```python
from build123d import *

# Parameters (mm, degrees)
BOSS_EXTRUDE1_DEPTH = 10
SKETCH4_R           = 2.5
CUT_EXTRUDE1_DEPTH  = 5
SKETCH5_R           = 2.5
CUT_EXTRUDE2_DEPTH  = 5


with BuildPart() as part:
    # 3DSketch1 → Boss-Extrude1 (new body)
    with BuildSketch(Plane(origin=(0, 0, 0), x_dir=(0.8320502943378437, 0.554700196225229, 0), z_dir=(0, 0, -1))):
        Polygon((0, 0), (8.320502943, 5.547001962), (13.867504906, -2.773500981), (18.027756377, 0), (9.707253434, 12.480754415), (-2.773500981, 4.160251472), align=None)
    extrude(amount=-BOSS_EXTRUDE1_DEPTH)

    # Sketch4 → Cut-Extrude1 (cut)
    with BuildSketch(Plane.ZY.offset(-10)):
        with Locations((5, 5)):
            Circle(SKETCH4_R)
    extrude(amount=-CUT_EXTRUDE1_DEPTH, mode=Mode.SUBTRACT)

    # Sketch5 → Cut-Extrude2 (cut)
    with BuildSketch(Plane(origin=(0, 0, 0), x_dir=(1, 0, 0), z_dir=(0, 1, 0))):
        with Locations(Location((5, -5, 0), (0, 0, 270))):
            Circle(SKETCH5_R)
    extrude(amount=-CUT_EXTRUDE2_DEPTH, mode=Mode.SUBTRACT)


solid = part.part
```
Input: part model. Units: mm. Frame: model coordinates. A direction names the side the tool comes from. Give positions to 0.01 mm unless a question says otherwise; leave off trailing zeros. Write each loop counter-clockwise with the first axis right and the second up, starting at its lowest first coordinate (ties: lowest second). Pieces come first, ordered by that corner, then holes. Notation, with made-up numbers: (31, -4) - (64, -4) arc R26 cw to (64, 28) - close; hole circle Ø6 at (-39.5, -29). An arc over 180 degrees is marked (long way). Write item = value, one per line. Start each with the question number.
1. First-contact query: pin 1 Ø5 at (y, z) = (4, 7) entering from -X; pin 2 Ø2 at (x, z) = (6.5, 3.5) entering from +Y; pin 3 Ø6 at (y, z) = (5, 5) entering from +X. Flat tips, straight axial feed; report the tip coordinate or a pass-through.
2. Section query B-B, the plane z = 5. Output: boundary loops of the cut face in (x, y), then the cut area to 3 significant figures.
3. Section query A-A, the plane x = 3. Output: boundary loops of the cut face in (y, z).
4. Section query C-C, the plane y = -2.25. Output: boundary loops of the cut face in (x, z), then the cut area to 3 significant figures.
5. Mould query, pull axis Z, two halves, no side actions, for faces 3 (the cylindrical face through (5.751, -2.465, 7.385)), 4 (the flat face through (12, 10, 5)), 5 (the cylindrical face through (12.465, 5.751, 7.385)), 6 (the flat face through (11, 1, 10)). Classes: released by +Z, released by -Z, zero draft, split by the parting line, or undercut.
6. Ray query, L1, parallel to X at y = -1.4, z = 5; L2, parallel to Y at x = 12.05, z = 5; L3, parallel to X at y = 8, z = 8.25. Return the intervals inside material, ascending.
7. Section query D-D, the plane y = 5. Output: boundary loops of the cut face in (x, z).
8. Access query for faces 1 (the flat face through (3, 0, 3)), 2 (the flat face through (0, -3, 5)). Directions: +Z, -Z, +X, -X, +Y, -Y. A direction counts if a zero-diameter tool reaches every point of the face in a straight line with its end or side. Return the directions, or none.
Check sheet entries:
q1.pin_1 = 10
q1.pin_2 = 0
q1.pin_3 = 15
q2.outline = (0, -5) - (2.5, -5) - (2.5, 0) - (0, 0) - close; (7.5, -5) - (15, -5) - (15, 2.5) - (10, 2.5) - (10, 0) - (7.5, 0) - close; (10, 7.5) - (15, 7.5) - (15, 10) - (10, 10) - close
q2.area = 75.0 mm2
q3.outline = (-5, 0) - (0, 0) - (0, 3.5) - (-5, 3.5) - close; (-5, 6.5) - (0, 6.5) - (0, 10) - (-5, 10) - close
q4.outline = (0, 0) - (15, 0) - (15, 10) - (0, 10) - close; hole circle Ø5 at (5, 5)
q4.area = 130 mm2
q5.face_3 = undercut
q5.face_4 = zero draft
q5.face_5 = undercut
q5.face_6 = released by +Z
q6.L1 = 0 to 2.5, 7.5 to 15
q6.L2 = -5 to 2.5, 7.5 to 10
q6.L3 = 10 to 15
q7.outline = (10, 0) - (15, 0) - (15, 2.5) - (10, 2.5) - close; (10, 7.5) - (15, 7.5) - (15, 10) - (10, 10) - close
q8.face_1 = +Z, -Z, -X, +Y
q8.face_2 = +Z, -Z, -X, +Y, -Y
